Autodesk Inventor part; units mm, degrees
ref_plane "YZ Plane" through (0, 0, 0) normal (1, 0, 0) x (0, 1, 0)
ref_plane "XZ Plane" through (0, 0, 0) normal (0, 1, 0) x (-1, 0, 0)
ref_plane "XY Plane" through (0, 0, 0) normal (0, 0, 1) x (1, 0, 0)
sketch "Sketch1" plane through (0, 0, 0) normal (0, 1, 0) x (-1, 0, 0)
  line L0 (32.6452, 15.2227) -> (29.9263, 13.9549)
  line L1 (-29.9263, 13.9549) -> (-32.6452, 15.2227)
  line L2 (36.02, 0) -> (-36.02, 0) construction
  arc A0 (29.9263, 13.9549) -> (-29.9263, 13.9549) centre (0, 0) ccw
  arc A1 (32.6452, 15.2227) -> (-32.6452, 15.2227) centre (0, 0) ccw
  dimension "d2" = 25
  dimension "d3" = 25
extrude "Extrusion1" add sketch "Sketch1" along normal blind 6
sketch "Sketch2" plane through (0, 0, 0) normal (0, -1, 0) x (1, 0, 0)
  arc A0 (32.6452, 15.2227) -> (-32.6452, 15.2227) centre (0, 0) ccw
  line L0 (2, 35.9644) -> (2, 42.9644)
  line L1 (2, 42.9644) -> (-2, 42.9644)
  line L2 (-2, 42.9644) -> (-2, 35.9644)
  dimension "d6" = 2
  dimension "d7" = 2
  dimension "d8" = 7
extrude "Extrusion2" add sketch "Sketch2" against normal blind 26
sketch "Sketch3" plane through (-2, 0, 35.9644) normal (-1, 0, 0) x (0, 0, 1)
  line L0 (7, 0) -> (7, 26)
  line L1 (7, 20) -> (-82.04, 20)
  line L2 (-82.04, 20) -> (-82.04, 26)
  line L3 (-82.04, 26) -> (-67.04, 41)
  line L4 (-67.04, 41) -> (-67.04, 69)
  line L5 (-67.04, 69) -> (-8, 69)
  line L6 (-8, 69) -> (-8, 41)
  line L7 (-8, 41) -> (7, 26)
  line L8 (-40.52, 59) -> (-27.52, 59)
  line L9 (-27.52, 59) -> (-27.52, 35)
  line L10 (-27.52, 35) -> (-40.52, 35)
  line L11 (-40.52, 35) -> (-40.52, 59)
  line L12 (7, 0) -> (0, 0)
  point P0 (-35.9644, 0)
  dimension "d11" = 15
  dimension "d12" = 15
  dimension "d13" = 89.04
  dimension "d14" = 24
  dimension "d15" = 13
  dimension "d16" = 19.52
  dimension "d17" = 10
  dimension "d18" = 15
  dimension "d19" = 15
  dimension "d20" = 15
  dimension "d21" = 20
  dimension "d22" = 6
extrude "Extrusion3" add sketch "Sketch3" along normal blind 4
sketch "Sketch4" plane through (-6, 0, 35.9644) normal (-1, 0, 0) x (0, 0, 1)
  line L0 (-40.52, 35) -> (-40.52, 59)
  line L1 (-27.52, 35) -> (-40.52, 35)
  line L2 (-27.52, 59) -> (-27.52, 35)
  line L3 (-40.52, 59) -> (-27.52, 59)
  line L4 (-46.52, 29) -> (-46.52, 65)
  line L5 (-46.52, 65) -> (-21.52, 65)
  line L6 (-21.52, 65) -> (-21.52, 29)
  line L7 (-21.52, 29) -> (-46.52, 29)
  point P0 (-35.9644, 0)
  dimension "d49" = 6
extrude "Extrusion4" add sketch "Sketch4" along normal blind 6
sketch "Sketch5" plane through (-2, 20, -46.0756) normal (0, -1, 0) x (1, 0, 0)
  line L0 (0, 82.04) -> (0, 89.04)
  line L1 (0, 82.04) -> (0, 89.04)
  line L2 (0, 89.04) -> (-4, 89.04)
  line L3 (0, 89.04) -> (-4, 89.04)
  line L4 (-4, 89.04) -> (-4, 81.54)
  line L5 (-4, 89.04) -> (-4, 74.04)
  arc A0 (0, 82.04) -> (-30.6452, 61.2983) centre (2, 46.0756) ccw
  point P0 (-4, 81.5923)
extrude "Extrusion5" add sketch "Sketch5" along normal up to surface (20 mm away)
sketch "Sketch6" plane through (-2, 0, 35.9644) normal (1, 0, 0) x (0, 0, -1)
  circle A0 centre (77.54, 24) radius 1.75
  circle A1 centre (62.04, 64) radius 1.75
  circle A2 centre (13, 64) radius 1.75
  line L0 (8, 69) -> (67.04, 69)
  line L1 (67.04, 69) -> (67.04, 41)
  line L2 (8, 41) -> (8, 69)
  line L3 (82.04, 20) -> (0, 20)
  line L4 (82.04, 26) -> (82.04, 20)
  point P0 (35.9644, 0)
  dimension "d36" = 3.5
  dimension "d37" = 3.5
  dimension "d38" = 3.5
  dimension "d40" = 5
  dimension "d41" = 5
  dimension "d42" = 5
  dimension "d43" = 5
  dimension "d44" = 4
  dimension "d45" = 4.5
extrude "Extrusion6" cut sketch "Sketch6" against normal blind 6
sketch "Sketch7" plane through (2, 0, 42.9644) normal (1, 0, 0) x (0, 0, -1)
  circle A0 centre (4, 23) radius 1.75
  line L0 (0, 0) -> (0, 26)
  line L1 (0, 26) -> (7, 26)
  point P0 (42.9644, 0)
  dimension "d50" = 3.5
  dimension "d51" = 4
  dimension "d52" = 3
extrude "Extrusion7" cut sketch "Sketch7" against normal through all
sketch "Sketch8" plane through (-2, 0, 35.9644) normal (1, 0, 0) x (0, 0, -1)
  line L0 (82.04, 20) -> (0, 20)
  line L1 (20, 22) -> (40, 22)
  line L2 (40, 22) -> (40, 20)
  line L3 (40, 20) -> (20, 20)
  line L4 (20, 20) -> (20, 22)
  line L5 (0, 6) -> (0, 26)
  line L6 (67.04, 20) -> (63.04, 20)
  line L7 (63.04, 20) -> (63.04, 24)
  line L8 (63.04, 24) -> (67.04, 24)
  line L9 (67.04, 24) -> (67.04, 20)
  line L10 (82.04, 26) -> (82.04, 20)
  point P0 (35.9644, 0)
  dimension "d55" = 2
  dimension "d56" = 20
  dimension "d57" = 20
  dimension "d60" = 4
  dimension "d61" = 4
  dimension "d62" = 15
extrude "Extrusion8" add sketch "Sketch8" along normal blind 4
sketch "Sketch10" plane through (-6, 0, 35.9644) normal (-1, 0, 0) x (0, 0, 1)
  circle A0 centre (-62.04, 64) radius 1.75
  circle A1 centre (-13, 64) radius 1.75
  circle A2 centre (-77.54, 24) radius 1.75
  circle A3 centre (3, 23) radius 1.75
  line L0 (-62.04, 60.8246) -> (-64.79, 62.4123)
  line L1 (-64.79, 62.4123) -> (-64.79, 65.5877)
  line L2 (-64.79, 65.5877) -> (-62.04, 67.1754)
  line L3 (-62.04, 67.1754) -> (-59.29, 65.5877)
  line L4 (-59.29, 65.5877) -> (-59.29, 62.4123)
  line L5 (-59.29, 62.4123) -> (-62.04, 60.8246)
  line L6 (-13, 60.8246) -> (-15.75, 62.4123)
  line L7 (-15.75, 62.4123) -> (-15.75, 65.5877)
  line L8 (-15.75, 65.5877) -> (-13, 67.1754)
  line L9 (-13, 67.1754) -> (-10.25, 65.5877)
  line L10 (-10.25, 65.5877) -> (-10.25, 62.4123)
  line L11 (-10.25, 62.4123) -> (-13, 60.8246)
  line L12 (-74.79, 25.5877) -> (-74.79, 22.4123)
  line L13 (-74.79, 22.4123) -> (-77.54, 20.8246)
  line L14 (-77.54, 20.8246) -> (-80.29, 22.4123)
  line L15 (-80.29, 22.4123) -> (-80.29, 25.5877)
  line L16 (-80.29, 25.5877) -> (-77.54, 27.1754)
  line L17 (-77.54, 27.1754) -> (-74.79, 25.5877)
  circle A4 centre (3, 23) radius 1.75
  line L18 (0.25, 24.5877) -> (3, 26.1754)
  line L19 (3, 26.1754) -> (5.75, 24.5877)
  line L20 (5.75, 24.5877) -> (5.75, 21.4123)
  line L21 (5.75, 21.4123) -> (3, 19.8246)
  line L22 (3, 19.8246) -> (0.25, 21.4123)
  line L23 (0.25, 21.4123) -> (0.25, 24.5877)
  line L24 (-67.04, 69) -> (-67.04, 41)
  line L25 (-8, 41) -> (-8, 69)
  line L26 (7, 26) -> (7, 0)
  line L27 (-82.04, 26) -> (-82.04, 20)
  point P0 (-35.9644, 0)
  dimension "d63" = 5.5
  dimension "d64" = 5.5
  dimension "d65" = 5.5
  dimension "d66" = 5.5
extrude "Extrusion9" cut sketch "Sketch10" against normal blind 2 contours A3 | L0 L1 L2 L3 L4 L5 | L6 L7 L8 L9 L10 L11 | L12 L13 L14 L15 L16 L17 | L18 L19 L20 L21 L22 L23
sketch "Sketch11" plane through (-12, 0, 35.9644) normal (-1, 0, 0) x (0, 0, 1)
  circle A0 centre (-34.02, 32.5) radius 0.5
  circle A1 centre (-34.02, 61.5) radius 0.5
  line L0 (-40.52, 59) -> (-27.52, 59)
  line L1 (-27.52, 35) -> (-40.52, 35)
  line L2 (-21.52, 29) -> (-21.52, 65)
  point P0 (-35.9644, 0)
  dimension "d69" = 2.5
  dimension "d70" = 2.5
  dimension "d71" = 12.5
  dimension "d72" = 12.5
  dimension "d73" = 1
  dimension "d74" = 1
extrude "Extrusion10" cut sketch "Sketch11" against normal blind 4
equation "\"d3\" = d2"
equation "\"d12\" = d11"
equation "\"d20\" = d19"
equation "\"d37\" = d36"
equation "\"d38\" = d36"
properties part number "_3DPrint"
For this review, take the finished solid that the model builds, in its own axes (mm). A direction names the side the tool comes from. Round coordinates to 2 decimals unless told otherwise and drop trailing zeros. Write each loop counter-clockwise with the first axis right and the second up, starting at its lowest first coordinate (ties: lowest second). Pieces come first, ordered by that corner, then holes. Notation, with made-up numbers: (-38.75, 8.5) - (-23.75, 8.5) arc R18 cw to (-23.75, 38.5) - close; hole circle Ø4 at (0.25, 34). An arc over 180 degrees is marked (long way). Write each question's results on one line, items separated by ' | '.
Item 1: For pin 1 (1.8 mm diameter, centred on x = -8.5, y = 53, fed in from -Z); pin 2 (2 mm diameter, centred on x = 1, y = 21.5, fed in from -Z); pin 3 (12 mm diameter, centred on y = 39.5, z = -28.5, fed in from +X); pin 4 (8 mm diameter, centred on x = -0.5, z = 0.5, fed in from +Y), all flat-tipped, find the tip position at first contact; note any pin that passes through.
Calculated:
pin 1: stops at z = -10.56 | pin 2: stops at z = -31.08 | pin 3: stops at x = -2 | pin 4: stops at y = 69
Item 2: Take a section at D-D on z = 12. State the section outline as (x, y) points.
Calculated:
outline: (-12, 29) - (-6, 29) - (-6, 20) - (2, 20) - (2, 22) - (-2, 22) - (-2, 69) - (-6, 69) - (-6, 65) - (-12, 65) - close
Item 3: Take a section at A-A on x = 0. State the section outline as (y, z) points.
Calculated:
outline: (0, 33.02) - (6, 33.02) - (6, 36.02) - (26, 36.02) - (26, 42.96) - (0, 42.96) - close; (20, -31.08) - (24, -31.08) - (24, -27.08) - (20, -27.08) - close; (20, -4.04) - (22, -4.04) - (22, 15.96) - (20, 15.96) - close; hole circle Ø3.5 at (23, 38.96)
Item 4: To check wall thickness, follow line 1 along Z through (x, y) = (-2.8, 64); line 2 along Z through (x, y) = (-11.5, 37.5); line 3 along X through (y, z) = (38, -7.5). State the ranges of each line that lie inside material, in increasing order. Write a range as from..to.
Calculated:
line 1: z = -31.08..-27.83, -24.33..21.21, 24.71..27.96 | line 2: z = -10.56..-4.56, 8.44..14.44 | line 3: x = -12..-2
Item 5: Draft analysis for pull direction X (two halves, no side actions). For faces 1 (the face through (2, 13, 39)), 2 (the face through (0.524, 2.958, 33.016)), 3 (the face through (0, 21, 15.964)), state which applies: pulls with the +X half, pulls with the -X half, needs draft (parallel to the pull), parting line crosses it, or undercut.
Calculated:
face 1: pulls with the +X half | face 2: undercut | face 3: needs draft
Item 6: For faces 4 (the face through (0, 26, 40)), 5 (the face through (-9, 47, -10.556)), 6 (the face through (-4, 55, 27.964)), 7 (the face through (-4, 64, -28)), 8 (the face through (0, 21, -4.036)), list the 3-axis set-ups (+Z, -Z, +X, -X, +Y, -Y) from which the entire face can be reached by the end or side of a thin tool; tool diameter is ignored.
Calculated:
face 4: +Z, -Z, +X, +Y | face 5: -Z, -X, +Y, -Y | face 6: +Z, +X, -X, +Y | face 7: -X | face 8: +X, +Y, -Y
Item 7: Take a section at C-C on z = -2.5. State the section outline as (x, y) points, then the cut area to 3 significant figures.
Calculated:
outline: (-12, 29) - (-6, 29) - (-6, 20) - (2, 20) - (2, 22) - (-2, 22) - (-2, 35) - (-12, 35) - close; (-12, 59) - (-2, 59) - (-2, 69) - (-6, 69) - (-6, 65) - (-12, 65) - close | area: 180 mm^2
Item 8: Take a section at B-B on y = 50. State the section outline as (x, z) points.
Calculated:
outline: (-12, -10.56) - (-6, -10.56) - (-6, -31.08) - (-2, -31.08) - (-2, -4.56) - (-12, -4.56) - close; (-12, 8.44) - (-2, 8.44) - (-2, 27.96) - (-6, 27.96) - (-6, 14.44) - (-12, 14.44) - close
